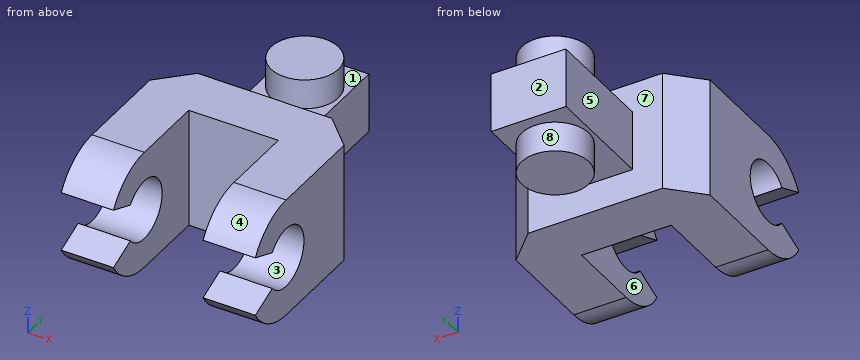
```python
from build123d import *

# Parameters (mm, degrees)
BOSS_EXTRUDE1_START = 6
SKETCH1_R           = 4
BOSS_EXTRUDE1_DEPTH = 7
BOSS_EXTRUDE2_START = -6
SKETCH1_2_R         = 4
BOSS_EXTRUDE2_DEPTH = 7
SKETCH2_W           = 26
SKETCH2_H           = 16
BOSS_EXTRUDE3_DEPTH = 7
CHAMFER1_SIZE       = 4
SKETCH3_W           = 10
SKETCH3_H           = 8
BOSS_EXTRUDE4_DEPTH = 15
SKETCH5_R           = 4.5
BOSS_EXTRUDE5_DEPTH = 8
CUT_EXTRUDE1_REACH  = 44


with BuildPart() as part:
    # Sketch1 → Boss-Extrude1 (new body)
    with BuildSketch(Plane(origin=(0, 0, 0), x_dir=(0, 0, -1), z_dir=(1, 0, 0)).offset(BOSS_EXTRUDE1_START)):
        with BuildLine():
            Line((-8, 0), (-8, 10))
            Line((-8, 10), (8, 10))
            Line((8, 10), (8, 0))
            ThreePointArc((8, 0), (0, -8), (-8, 0))
        make_face()
        Circle(SKETCH1_R, mode=Mode.SUBTRACT)
    extrude(amount=BOSS_EXTRUDE1_DEPTH)



with BuildPart() as body_2:
    # Sketch1<2> → Boss-Extrude2 (new body)
    with BuildSketch(Plane(origin=(0, 0, 0), x_dir=(0, 0, -1), z_dir=(1, 0, 0)).offset(BOSS_EXTRUDE2_START)):
        with BuildLine():
            Line((-8, 0), (-8, 10))
            Line((-8, 10), (8, 10))
            Line((8, 10), (8, 0))
            ThreePointArc((8, 0), (0, -8), (-8, 0))
        make_face()
        Circle(SKETCH1_2_R, mode=Mode.SUBTRACT)
    extrude(amount=-BOSS_EXTRUDE2_DEPTH)


with BuildPart() as part_1:
    add(part.part)

    add(body_2.part)  # Boss-Extrude3 merges body 2
    # Sketch2 → Boss-Extrude3 (add)
    with BuildSketch(Plane(origin=(0, 10, 0), x_dir=(1, 0, 0), z_dir=(0, 1, 0))):
        Rectangle(SKETCH2_W, SKETCH2_H)
    extrude(amount=BOSS_EXTRUDE3_DEPTH)

    # Chamfer1
    chamfer1_edges = [part_1.edges().sort_by_distance(p)[0] for p in [
        (-13, 17, 0),
        (13, 17, 0),
    ]]
    chamfer(chamfer1_edges, length=CHAMFER1_SIZE)

    # Sketch3 → Boss-Extrude4 (add)
    with BuildSketch(Plane(origin=(0, 17, 0), x_dir=(1, 0, 0), z_dir=(0, 1, 0))):
        Rectangle(SKETCH3_W, SKETCH3_H)
    extrude(amount=BOSS_EXTRUDE4_DEPTH)

    # Sketch5 → Boss-Extrude5 (add, symmetric)
    with BuildSketch(Plane.XY):
        with Locations(Location((0, 26, 0), (0, 0, 180))):
            Circle(SKETCH5_R)
    extrude(amount=BOSS_EXTRUDE5_DEPTH, both=True)

    # Cut-Extrude1: up to this face of the body (flat: up to its plane)
    cut_extrude1_end = Plane(part_1.part.faces().sort_by_distance((13, 6.5, 7.735992424))[0])
    # Sketch6 → Cut-Extrude1 (cut, up to the picked face)
    with BuildSketch(Plane.ZY.offset(13), mode=Mode.PRIVATE) as cut_extrude1_sk1:
        with BuildLine():
            Line((-2.488370132, -3.13177491), (-4, -6.92820323))
            ThreePointArc((-4, -6.92820323), (0, -8), (4, -6.92820323))
            Line((4, -6.92820323), (2.488370132, -3.13177491))
            ThreePointArc((2.488370132, -3.13177491), (0, -4), (-2.488370132, -3.13177491))
        make_face()
    cut_extrude1_tool1 = split(extrude(cut_extrude1_sk1.sketch, amount=-CUT_EXTRUDE1_REACH, mode=Mode.PRIVATE), bisect_by=cut_extrude1_end, keep=Keep.BOTH, mode=Mode.PRIVATE)
    add(cut_extrude1_tool1.solids().sort_by(Axis((-13, -5.819668, 0), (1, 0, 0)))[0], mode=Mode.SUBTRACT)


solid = part_1.part
```
Source: CAD feature listing. Evaluate the final solid. Frame: model axes, mm. Face numbers are marked on the shaded views. A direction names the side the tool comes from. Round coordinates to 2 decimals unless told otherwise and drop trailing zeros. Loops run counter-clockwise (first coordinate to the right, second up) from the corner with the lowest first, then second, coordinate; pieces in that order, holes last. Notation, with made-up numbers: M -24,3.5 L -5,3.5 A27 ccw -5,32.5 Z; hole C 49.25,62.25 d1. An arc over 180 degrees is marked long. Use a Markdown table: item, result. Add a question column.
1. Cut plane D-D, the plane y = 26. Output: boundary loops of the cut face in (x, z), and give its area (3 significant figures).
2. Ray query, line 1 along X through (y, z) = (8, 6.25); line 2 along Z through (x, y) = (9.25, 0); line 3 along Y through (x, z) = (-1.5, -0.5). Return the intervals inside material, ascending. Write a range as [from, to].
3. Cut plane A-A, the plane x = 0. Output: boundary loops of the cut face in (y, z), and give its area (3 significant figures).
4. Cut plane C-C, the plane z = 0. Output: boundary loops of the cut face in (x, y).
5. Cut plane B-B, the plane y = 0.5. Output: boundary loops of the cut face in (x, z), and give its area (3 significant figures).
6. Set-up query: the marked faces 5, 6, 7 and 8. Return all of +Z, -Z, +X, -X, +Y, -Y with unobstructed straight access to the full face (end or side cutting, diameter ignored); none if empty.
7. Pull-direction query (Y, two-part tool) for the marked faces 1, 2, 3 and 4; classes: +Y half, -Y half, draft (parallel to the pull), parting line (faces both ways), or undercut.
8. Contact query for flat-ended pins moving along their axis: pin 1 (6 mm diameter, centred on y = 24.5, z = -4.5, fed in from +X); pin 2 (4 mm diameter, centred on y = 24, z = 1, fed in from -X). Output: stop coordinate, or through.
Solution:
| question | item | result |
|---|---|---|
| 1 | outline | M -5,-4 L -4.5,-4 L -4.5,-8 L 4.5,-8 L 4.5,-4 L 5,-4 L 5,4 L 4.5,4 L 4.5,8 L -4.5,8 L -4.5,4 L -5,4 Z |
| 1 | area | 152 mm2 |
| 2 | line 1 | x = [-13, -6], [6, 13] |
| 2 | line 2 | z = [-8, -4], [4, 8] |
| 2 | line 3 | y = [10, 32] |
| 3 | outline | M 10,-8 L 17,-8 L 17,-4 L 21.5,-4 L 21.5,-8 L 30.5,-8 L 30.5,-4 L 32,-4 L 32,4 L 30.5,4 L 30.5,8 L 21.5,8 L 21.5,4 L 17,4 L 17,8 L 10,8 Z |
| 3 | area | 304 mm2 |
| 4 | outline | M -13,4 L -6,4 L -6,10 L 6,10 L 6,4 L 13,4 L 13,13 L 9,17 L 5,17 L 5,32 L -5,32 L -5,17 L -9,17 L -13,13 Z |
| 5 | outline | M -13,-8 L -6,-8 L -6,-3.97 L -13,-3.97 Z; M -13,3.97 L -6,3.97 L -6,8 L -13,8 Z; M 6,-8 L 13,-8 L 13,-3.97 L 6,-3.97 Z; M 6,3.97 L 13,3.97 L 13,8 L 6,8 Z |
| 5 | area | 113 mm2 |
| 6 | face 5 | +Z, -Z, -X, +Y |
| 6 | face 6 | +Z, -Z, -Y |
| 6 | face 7 | none |
| 6 | face 8 | -Z |
| 7 | face 1 | undercut |
| 7 | face 2 | +Y half |
| 7 | face 3 | undercut |
| 7 | face 4 | -Y half |
| 8 | pin 1 | stops at x = 5 |
| 8 | pin 2 | stops at x = -5 |
